Geometry: final body of the model. Coordinates: model frame, mm. Round coordinates to 2 decimals unless told otherwise and drop trailing zeros. Loops run counter-clockwise (first coordinate to the right, second up) from the corner with the lowest first, then second, coordinate; pieces in that order, holes last. Notation, with made-up numbers: (-33, 30) -> (1, 30) arc R29 ccw to (1, 54) -> close; hole circle Ø1 at (-10, -5). An arc over 180 degrees is marked (long way). Answer in a Markdown table with one row per item.
```python
from build123d import *

# Parameters (mm, degrees)
F1_DEPTH = 12
F3_DEPTH = 25


with BuildPart() as f1:
    # F0 (on Top) → F1 (new body)
    with BuildSketch(Plane.XY):
        Polygon((320, 250), (-320, 250), (-320, 21.803056), (-320, -88.196944), (-320, -250), (320, -250), align=None)
    extrude(amount=F1_DEPTH)

    # F2 (on face) → F3 (cut)
    with BuildSketch(Plane.XY.offset(12)):
        Polygon((-320, 60), (-180, 250), (-320, 250), align=None)
        Polygon((-320, -250), (-180, -250), (-320, -60), align=None)
    extrude(amount=-F3_DEPTH, mode=Mode.SUBTRACT)


solid = f1.part
```
Item 1: Line query: probe 1 along X at (y, z) = (-155, 9.5); probe 2 along Y at (x, z) = (-253, 3.25); probe 3 along X at (y, z) = (221, 9.5). Output: solid intervals per line, ascending. Write a range as [from, to].
Answer:
| item | result |
|---|---|
| probe 1 | x = [-250, 320] |
| probe 2 | y = [-150.93, 150.93] |
| probe 3 | x = [-201.37, 320] |
Item 2: Pin query (flat end, axial travel): pin 1 Ø1 at (y, z) = (137, 8) entering from -X; pin 2 Ø1 at (y, z) = (166, 2.5) entering from -X. Return the tip coordinate at first contact, or that it passes through.
Answer:
| item | result |
|---|---|
| pin 1 | stops at x = -263.63 |
| pin 2 | stops at x = -242.26 |
Item 3: Cut plane C-C (y = -212). Output: boundary loops of the cut face in (x, z).
Answer:
| item | result |
|---|---|
| outline | (-208, 0) -> (320, 0) -> (320, 12) -> (-208, 12) -> close |
Item 4: Cut plane A-A (z = 4.5). Output: boundary loops of the cut face in (x, y).
Answer:
| item | result |
|---|---|
| outline | (-320, -60) -> (-180, -250) -> (320, -250) -> (320, 250) -> (-180, 250) -> (-320, 60) -> close |
Item 5: Draft query along X for faces 1 (the face through (-250.98, 153.67, 6.08)), 2 (the face through (-4, 3, 12)). Return one class per face: pulls with the +X half, pulls with the -X half, needs draft (parallel to the pull), parting line crosses it, or undercut.
Answer:
| item | result |
|---|---|
| face 1 | pulls with the -X half |
| face 2 | needs draft |
Item 6: Cut plane B-B (x = -229). Output: boundary loops of the cut face in (y, z).
Answer:
| item | result |
|---|---|
| outline | (-183.5, 0) -> (183.5, 0) -> (183.5, 12) -> (-183.5, 12) -> close |
